Part print with two shaded views. Sizes in mm from the minimum x, y, z corner. A direction names the side the tool comes from. Give positions to 0.01 mm unless a question says otherwise; leave off trailing zeros. Write each loop counter-clockwise with the first axis right and the second up, starting at its lowest first coordinate (ties: lowest second). Pieces come first, ordered by that corner, then holes. Notation, with made-up numbers: (-20.5, -39.75) -> (-11.5, -39.75) arc R7 ccw to (-11.5, -29.75) -> close; hole circle Ø9 at (-3, 31). An arc over 180 degrees is marked (long way). Answer as a JSON object with one key per item and string values.
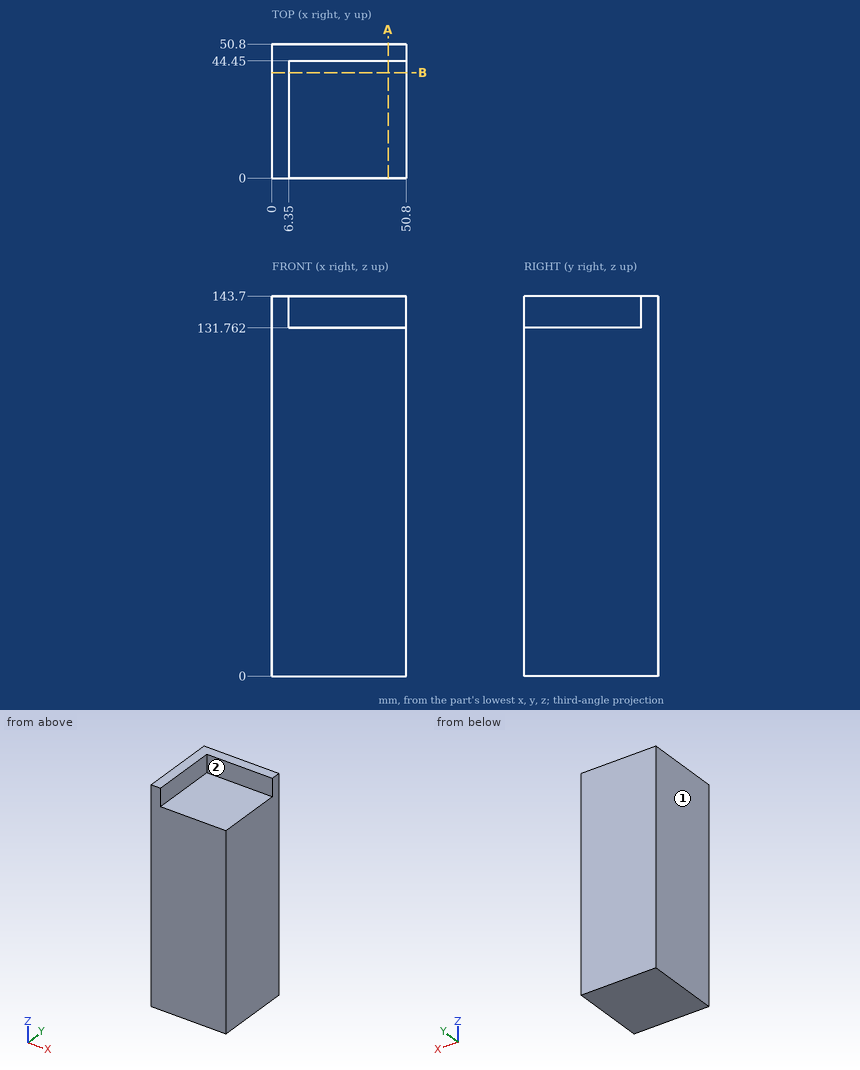
1) Slice it at A-A (x = 44). List the corners of the cut face in (y, z).
Model answer:
{"outline": "(0, 0) -> (50.8, 0) -> (50.8, 143.7) -> (44.45, 143.7) -> (44.45, 131.76) -> (0, 131.76) -> close"}
2) Wall check: probe 1 along Z at (x, y) = (14, 41.5); probe 2 along X at (y, z) = (42, 136); probe 3 along Y at (x, z) = (8, 136.5). Give the ranges that are in metal, low to high.
Model answer:
{"probe 1": "z = 0 to 131.76", "probe 2": "x = 0 to 6.35", "probe 3": "y = 44.45 to 50.8"}
3) 3-axis set-ups, long thin cutter, end or side, ignore diameter. For the marked faces 1 and 2: which of +Z, -Z, +X, -X, +Y, -Y reach the whole face in a straight line?
Model answer:
{"face 1": "+Z, -Z, -X, +Y, -Y", "face 2": "+Z, +X, -Y"}
4) Slice it at B-B (y = 40). List the corners of the cut face in (x, z), then the cut area to 3 significant figures.
Model answer:
{"outline": "(0, 0) -> (50.8, 0) -> (50.8, 131.76) -> (6.35, 131.76) -> (6.35, 143.7) -> (0, 143.7) -> close", "area": "6,770 mm2"}
5) Pin check, flat tips, straight feed: pin 1 (3 mm diameter, centred on x = 44.5, y = 30, fed in from +Z); pin 2 (3 mm diameter, centred on x = 10, y = 21, fed in from -Z); pin 3 (6 mm diameter, centred on x = 20, z = 135.5, fed in from -Y); pin 4 (13 mm diameter, centred on y = 17, z = 140.5, fed in from +X). Stop position of each tip, or through.
Model answer:
{"pin 1": "stops at z = 131.76", "pin 2": "stops at z = 0", "pin 3": "stops at y = 44.45", "pin 4": "stops at x = 6.35"}
